Here's how the part is built. I have some questions about the finished solid (model axes, mm). A direction names the side the tool comes from. Give positions to 0.01 mm unless a question says otherwise; leave off trailing zeros. Use a Markdown table: item, result.
```python
from build123d import *

# Parameters (mm, degrees)
F0_W     = 0.6829528259
F0_H     = 4.5069622906
F0_H_2   = 6.3992285019
F0_R     = 1.4814772489
F1_DEPTH = 2


with BuildPart() as f1:
    # F0 (on Front) → F1 (new body)
    with BuildSketch(Plane.XZ):
        with BuildLine():
            Line((15.6519781798, 28.567796193), (-34.3480218202, 28.567796193))
            Line((-34.3480218202, 28.567796193), (-34.3480218202, 18.567796193))
            Line((-34.3480218202, 18.567796193), (15.6519781798, 18.567796193))
            ThreePointArc((15.6519781798, 18.567796193), (20.6519781798, 23.567796193), (15.6519781798, 28.567796193))
        make_face()
        with BuildLine():
            add(Edge.make_bspline(
                [(-12.0378659954, 20.6372455488), (-12.3602618381, 20.5688186761), (-12.8168796234, 20.5688186761)],
                knots=[0, 0, 0, 1, 1, 1], degree=2))
            add(Edge.make_bspline(
                [(-12.8168796234, 20.5688186761), (-13.8156487851, 20.5688186761), (-14.3939874498, 21.1780810237)],
                knots=[0, 0, 0, 1, 1, 1], degree=2))
            add(Edge.make_bspline(
                [(-14.3939874498, 21.1780810237), (-14.9723261145, 21.7873433713), (-14.9723261145, 22.8676984197)],
                knots=[0, 0, 0, 1, 1, 1], degree=2))
            add(Edge.make_bspline(
                [(-14.9723261145, 22.8676984197), (-14.9723261145, 23.9585806792), (-14.4354383439, 24.6000826111)],
                knots=[0, 0, 0, 1, 1, 1], degree=2))
            add(Edge.make_bspline(
                [(-14.4354383439, 24.6000826111), (-13.8985505732, 25.2415845429), (-12.9932104109, 25.2415845429)],
                knots=[0, 0, 0, 1, 1, 1], degree=2))
            add(Edge.make_bspline(
                [(-12.9932104109, 25.2415845429), (-12.1470858115, 25.2415845429), (-11.653622787, 24.6843003006)],
                knots=[0, 0, 0, 1, 1, 1], degree=2))
            add(Edge.make_bspline(
                [(-11.653622787, 24.6843003006), (-11.1601597625, 24.1270160582), (-11.1601597625, 23.2137804875)],
                knots=[0, 0, 0, 1, 1, 1], degree=2))
            Line((-11.1601597625, 23.2137804875), (-11.1601597625, 22.7821648287))
            Line((-11.1601597625, 22.7821648287), (-14.264371162, 22.7821648287))
            add(Edge.make_bspline(
                [(-14.264371162, 22.7821648287), (-14.2433167396, 21.9886762853), (-13.8630212354, 21.5774570982)],
                knots=[0, 0, 0, 1, 1, 1], degree=2))
            add(Edge.make_bspline(
                [(-13.8630212354, 21.5774570982), (-13.4827257312, 21.1662379111), (-12.7918774969, 21.1662379111)],
                knots=[0, 0, 0, 1, 1, 1], degree=2))
            add(Edge.make_bspline(
                [(-12.7918774969, 21.1662379111), (-12.0641840234, 21.1662379111), (-11.3535972681, 21.4702111342)],
                knots=[0, 0, 0, 1, 1, 1], degree=2))
            Line((-11.3535972681, 21.4702111342), (-11.3535972681, 20.8609487866))
            add(Edge.make_bspline(
                [(-11.3535972681, 20.8609487866), (-11.7154701527, 20.7056724216), (-12.0378659954, 20.6372455488)],
                knots=[0, 0, 0, 1, 1, 1], degree=2))
        make_face(mode=Mode.SUBTRACT)
        Polygon((-10.5587928233, 20.6517204642), (-8.9099683707, 22.9584956162), (-10.4772069365, 25.1586827548), (-9.6995092099, 25.1586827548), (-8.5112502469, 23.4322201197), (-7.326938988, 25.1586827548), (-6.5571366698, 25.1586827548), (-8.1243752356, 22.9584956162), (-6.4755507831, 20.6517204642), (-7.2479849041, 20.6517204642), (-8.5112502469, 22.4781916056), (-9.7863587022, 20.6517204642), align=None, mode=Mode.SUBTRACT)
        with Locations((-5.2418932218, 22.9052016095)):
            Rectangle(F0_W, F0_H, mode=Mode.SUBTRACT)
        with BuildLine():
            add(Edge.make_bspline(
                [(-0.8277019798, 22.6255725623), (-0.5460990805, 22.3294947476), (-0.5460990805, 21.8807723706)],
                knots=[0, 0, 0, 1, 1, 1], degree=2))
            add(Edge.make_bspline(
                [(-0.5460990805, 21.8807723706), (-0.5460990805, 21.251771502), (-1.0145599784, 20.9102950891)],
                knots=[0, 0, 0, 1, 1, 1], degree=2))
            add(Edge.make_bspline(
                [(-1.0145599784, 20.9102950891), (-1.4830208763, 20.5688186761), (-2.3304613771, 20.5688186761)],
                knots=[0, 0, 0, 1, 1, 1], degree=2))
            add(Edge.make_bspline(
                [(-2.3304613771, 20.5688186761), (-3.2265902296, 20.5688186761), (-3.7279486625, 20.8530533782)],
                knots=[0, 0, 0, 1, 1, 1], degree=2))
            Line((-3.7279486625, 20.8530533782), (-3.7279486625, 21.486001951))
            add(Edge.make_bspline(
                [(-3.7279486625, 21.486001951), (-3.4029210171, 21.3215142762), (-3.0311788719, 21.2274273262)],
                knots=[0, 0, 0, 1, 1, 1], degree=2))
            add(Edge.make_bspline(
                [(-3.0311788719, 21.2274273262), (-2.6594367268, 21.1333403762), (-2.3133546589, 21.1333403762)],
                knots=[0, 0, 0, 1, 1, 1], degree=2))
            add(Edge.make_bspline(
                [(-2.3133546589, 21.1333403762), (-1.7790986911, 21.1333403762), (-1.4915742354, 21.3037496073)],
                knots=[0, 0, 0, 1, 1, 1], degree=2))
            add(Edge.make_bspline(
                [(-1.4915742354, 21.3037496073), (-1.2040497798, 21.4741588384), (-1.2040497798, 21.8241886105)],
                knots=[0, 0, 0, 1, 1, 1], degree=2))
            add(Edge.make_bspline(
                [(-1.2040497798, 21.8241886105), (-1.2040497798, 22.0873688902), (-1.4317007218, 22.2742268888)],
                knots=[0, 0, 0, 1, 1, 1], degree=2))
            add(Edge.make_bspline(
                [(-1.4317007218, 22.2742268888), (-1.6593516638, 22.4610848875), (-2.3225659687, 22.7163697588)],
                knots=[0, 0, 0, 1, 1, 1], degree=2))
            add(Edge.make_bspline(
                [(-2.3225659687, 22.7163697588), (-2.9515668373, 22.9506002078), (-3.2167209691, 23.1256150938)],
                knots=[0, 0, 0, 1, 1, 1], degree=2))
            add(Edge.make_bspline(
                [(-3.2167209691, 23.1256150938), (-3.481875101, 23.3006299798), (-3.6114913888, 23.5223593655)],
                knots=[0, 0, 0, 1, 1, 1], degree=2))
            add(Edge.make_bspline(
                [(-3.6114913888, 23.5223593655), (-3.7411076765, 23.7440887512), (-3.7411076765, 24.0520096785)],
                knots=[0, 0, 0, 1, 1, 1], degree=2))
            add(Edge.make_bspline(
                [(-3.7411076765, 24.0520096785), (-3.7411076765, 24.6033723646), (-3.2923852996, 24.9224784537)],
                knots=[0, 0, 0, 1, 1, 1], degree=2))
            add(Edge.make_bspline(
                [(-3.2923852996, 24.9224784537), (-2.8436629226, 25.2415845429), (-2.0633333932, 25.2415845429)],
                knots=[0, 0, 0, 1, 1, 1], degree=2))
            add(Edge.make_bspline(
                [(-2.0633333932, 25.2415845429), (-1.3356399197, 25.2415845429), (-0.6395280798, 24.9455067282)],
                knots=[0, 0, 0, 1, 1, 1], degree=2))
            Line((-0.6395280798, 24.9455067282), (-0.8829698385, 24.390196338))
            add(Edge.make_bspline(
                [(-0.8829698385, 24.390196338), (-1.5606590589, 24.6691674345), (-2.1120217449, 24.6691674345)],
                knots=[0, 0, 0, 1, 1, 1], degree=2))
            add(Edge.make_bspline(
                [(-2.1120217449, 24.6691674345), (-2.5975893611, 24.6691674345), (-2.8443208733, 24.5171808229)],
                knots=[0, 0, 0, 1, 1, 1], degree=2))
            add(Edge.make_bspline(
                [(-2.8443208733, 24.5171808229), (-3.0910523856, 24.3651942114), (-3.0910523856, 24.0980662275)],
                knots=[0, 0, 0, 1, 1, 1], degree=2))
            add(Edge.make_bspline(
                [(-3.0910523856, 24.0980662275), (-3.0910523856, 23.9164718344), (-2.998281337, 23.7894873495)],
                knots=[0, 0, 0, 1, 1, 1], degree=2))
            add(Edge.make_bspline(
                [(-2.998281337, 23.7894873495), (-2.9055102884, 23.6625028645), (-2.7002296702, 23.5473614921)],
                knots=[0, 0, 0, 1, 1, 1], degree=2))
            add(Edge.make_bspline(
                [(-2.7002296702, 23.5473614921), (-2.494949052, 23.4322201197), (-1.9106888309, 23.2137804875)],
                knots=[0, 0, 0, 1, 1, 1], degree=2))
            add(Edge.make_bspline(
                [(-1.9106888309, 23.2137804875), (-1.1093048791, 22.921650377), (-0.8277019798, 22.6255725623)],
                knots=[0, 0, 0, 1, 1, 1], degree=2))
        make_face(mode=Mode.SUBTRACT)
        Polygon((-17.5751790812, 20.6517204642), (-18.2989248505, 20.6517204642), (-19.0476727463, 22.5637251966), (-21.4570882074, 22.5637251966), (-22.1966247934, 20.6517204642), (-22.904579746, 20.6517204642), (-20.5280618199, 26.6890760815), (-19.9398538947, 26.6890760815), align=None, mode=Mode.SUBTRACT)
        with Locations((-16.5099568989, 23.8513347152)):
            Rectangle(F0_W, F0_H_2, mode=Mode.SUBTRACT)
        with Locations((17.7988428622, 23.567796193)):
            Circle(F0_R, mode=Mode.SUBTRACT)
        with BuildLine():
            add(Edge.make_bspline(
                [(-5.5261279239, 26.0363889878), (-5.6412692963, 26.149556508), (-5.6412692963, 26.3798392528)],
                knots=[0, 0, 0, 1, 1, 1], degree=2))
            add(Edge.make_bspline(
                [(-5.6412692963, 26.3798392528), (-5.6412692963, 26.6140697018), (-5.5261279239, 26.7232895179)],
                knots=[0, 0, 0, 1, 1, 1], degree=2))
            add(Edge.make_bspline(
                [(-5.5261279239, 26.7232895179), (-5.4109865515, 26.832509334), (-5.2372875669, 26.832509334)],
                knots=[0, 0, 0, 1, 1, 1], degree=2))
            add(Edge.make_bspline(
                [(-5.2372875669, 26.832509334), (-5.072799892, 26.832509334), (-4.9537108154, 26.7213156658)],
                knots=[0, 0, 0, 1, 1, 1], degree=2))
            add(Edge.make_bspline(
                [(-4.9537108154, 26.7213156658), (-4.8346217389, 26.6101219976), (-4.8346217389, 26.3798392528)],
                knots=[0, 0, 0, 1, 1, 1], degree=2))
            add(Edge.make_bspline(
                [(-4.8346217389, 26.3798392528), (-4.8346217389, 26.149556508), (-4.9537108154, 26.0363889878)],
                knots=[0, 0, 0, 1, 1, 1], degree=2))
            add(Edge.make_bspline(
                [(-4.9537108154, 26.0363889878), (-5.072799892, 25.9232214675), (-5.2372875669, 25.9232214675)],
                knots=[0, 0, 0, 1, 1, 1], degree=2))
            add(Edge.make_bspline(
                [(-5.2372875669, 25.9232214675), (-5.4109865515, 25.9232214675), (-5.5261279239, 26.0363889878)],
                knots=[0, 0, 0, 1, 1, 1], degree=2))
        make_face(mode=Mode.SUBTRACT)
    extrude(amount=F1_DEPTH)


solid = f1.part
```
Item 1: For faces 4 (the flat face through (-9.114, -0.986, 24.308)), 5 (the flat face through (-7, 0, 24)), which set-ups out of +Z, -Z, +X, -X, +Y, -Y let a thin tool reach every point of the face, with its end or its side?
Values:
| item | result |
|---|---|
| face 4 | +Y, -Y |
| face 5 | +Z, -Z, +X, -X, +Y |
Item 2: If we section it at A-A, the plane y = -0.5: Count the separate pieces of the cut face and the enclosed holes in it, plus the area to 3 significant figures.
Values:
| item | result |
|---|---|
| separate pieces | 1 |
| enclosed holes | 8 |
| area | 489 mm2 |
Item 3: Will this pin go through, and if not, where does the flat tip stop? pin 1 Ø3 at (x, z) = (4, 27) entering from +Y.
Values:
| item | result |
|---|---|
| pin 1 | stops at y = 0 |
Item 4: I need wall thicknesses on line 1 along X through (y, z) = (-0.5, 25.75); line 2 along X through (y, z) = (-1.35, 26); line 3 along Z through (x, y) = (-3, -0.4). Which ranges of each line are inside material? Lowest first, please. Write a range as [from, to].
Values:
| item | result |
|---|---|
| line 1 | x = [-34.35, -20.9], [-19.57, -16.85], [-16.17, 20.15] |
| line 2 | x = [-34.35, -20.8], [-19.67, -16.85], [-16.17, -5.48], [-5, 20.02] |
| line 3 | z = [18.57, 20.62], [21.22, 23], [23.79, 24.38], [25.08, 28.57] |
Item 5: Thinking about a two-plate mould opening in Z: for faces 1 (the cylindrical face through (20.65, -0.99, 23.46)), 2 (the flat face through (-34.348, -1, 24)), 3 (the flat face through (-9.746, -0.986, 21.789)), which applies, +Z half, -Z half, draft (parallel to the pull), parting line (faces both ways), or undercut?
Values:
| item | result |
|---|---|
| face 1 | parting line |
| face 2 | draft |
| face 3 | undercut |
